from build123d import *

# Parameters (mm, degrees)
ESQUISSE1_W             = 47
ESQUISSE1_H             = 25
BOSS_EXTRU_1_DEPTH      = 5
ESQUISSE2_W             = 4
ESQUISSE2_H             = 4
ENL_V_MAT_EXTRU_1_DEPTH = 5
ESQUISSE4_W             = 47
ESQUISSE4_H             = 12
BOSS_EXTRU_2_DEPTH      = 3
ESQUISSE5_R             = 3
ENL_V_MAT_EXTRU_2_DEPTH = 63


with BuildPart() as part:
    # Esquisse1 → Boss.-Extru.1 (new body)
    with BuildSketch(Plane.XY):
        with Locations((-12.5, -7.5)):
            Rectangle(ESQUISSE1_W, ESQUISSE1_H)
    extrude(amount=BOSS_EXTRU_1_DEPTH)

    # Esquisse2 → Enlèv. mat.-Extru.1 (cut)
    with BuildSketch(Plane.XY.offset(5)):
        with Locations((-25.3, -16)):
            Rectangle(ESQUISSE2_W, ESQUISSE2_H)
        with Locations((-25.3, 1)):
            Rectangle(ESQUISSE2_W, ESQUISSE2_H)
        with Locations((0.3, 1)):
            Rectangle(ESQUISSE2_W, ESQUISSE2_H)
        with Locations((0.3, -16)):
            Rectangle(ESQUISSE2_W, ESQUISSE2_H)
    extrude(amount=-ENL_V_MAT_EXTRU_1_DEPTH, mode=Mode.SUBTRACT)

    # Esquisse4 → Boss.-Extru.2 (add)
    with BuildSketch(Plane.XY.offset(5)):
        with Locations((-12.5, -7.5)):
            Rectangle(ESQUISSE4_W, ESQUISSE4_H)
    extrude(amount=BOSS_EXTRU_2_DEPTH)

    # Esquisse5 → Enlèv. mat.-Extru.2 (cut)
    with BuildSketch(Plane(origin=(11, 0, 0), x_dir=(0, 0, -1), z_dir=(1, 0, 0))):
        with Locations((-8, -7.5)):
            Circle(ESQUISSE5_R)
    extrude(amount=-ENL_V_MAT_EXTRU_2_DEPTH, mode=Mode.SUBTRACT)


solid = part.part
CAD build for the part. Positions are in the model's coordinates, mm. A direction names the side the tool comes from. Round coordinates to 2 decimals unless told otherwise and drop trailing zeros. Loops run counter-clockwise (first coordinate to the right, second up) from the corner with the lowest first, then second, coordinate; pieces in that order, holes last.
(1) Cut at A-A (y = 1). Give the cut face in (x, z).
(2) Cut at C-C (z = 7). Give the cut face in (x, y).
(3) Which spindle directions (+Z, -Z, +X, -X, +Y, -Y) get a long thin tool onto all of the face, cutting with end or side? Do faces 3 (the flat face through (-13, -13.5, 6)), 4 (the flat face through (-13, 2, 5)), 5 (the flat face through (-27.3, -16, 3)). Say none if no direction does.
(4) Cut at D-D (x = 3.5). Give the cut face in (y, z), plus the area to 3 significant figures.
(5) Cut at B-B (z = 1.25). Give the cut face in (x, y), plus the area to 3 significant figures.
(6) Two-plate mould, pull along X, no slides. Class faces 1 (the flat face through (2.3, -16, 3)), 2 (the flat face through (-13, -12, 8)): +X half, -X half, draft (parallel to the pull), parting line (faces both ways), or undercut.
(7) Drop flat-ended pins along their axis: pin 1 (1.5 mm diameter, centred on x = -6.5, z = 6, fed in from +Y); pin 2 (5 mm diameter, centred on x = -8, y = 3, fed in from +Z). Give the stop position or say it passes through.
(8) Wall check: line 1 along X through (y, z) = (2.25, 2.25); line 2 along Z through (x, y) = (7.5, 0); line 3 along Y through (x, z) = (-25, 6). Give the ranges that are in metal, low to high.
Findings below:
1. outline: (-36, 0) - (-27.3, 0) - (-27.3, 5) - (-36, 5) - close; (-23.3, 0) - (-1.7, 0) - (-1.7, 5) - (-23.3, 5) - close; (2.3, 0) - (11, 0) - (11, 5) - (2.3, 5) - close
2. outline: (-36, -13.5) - (11, -13.5) - (11, -10.33) - (-36, -10.33) - close; (-36, -4.67) - (11, -4.67) - (11, -1.5) - (-36, -1.5) - close
3. face 3: +Z, +X, -X, -Y
3. face 4: +Z, +X, -X, +Y
3. face 5: +Z, -Z
4. outline: (-20, 0) - (5, 0) - (5, 5) - (-1.5, 5) - (-1.5, 8) - (-4.5, 8) arc R3 cw to (-10.5, 8) - (-13.5, 8) - (-13.5, 5) - (-20, 5) - close
4. area: 147 mm2
5. outline: (-36, -20) - (11, -20) - (11, 5) - (-36, 5) - close; hole (-27.3, -18) - (-23.3, -18) - (-23.3, -14) - (-27.3, -14) - close; hole (-27.3, -1) - (-23.3, -1) - (-23.3, 3) - (-27.3, 3) - close; hole (-1.7, -18) - (2.3, -18) - (2.3, -14) - (-1.7, -14) - close; hole (-1.7, -1) - (2.3, -1) - (2.3, 3) - (-1.7, 3) - close
5. area: 1,110 mm2
6. face 1: undercut
6. face 2: draft
7. pin 1: stops at y = -1.5
7. pin 2: stops at z = 5
8. line 1: x = -36 to -27.3, -23.3 to -1.7, 2.3 to 11
8. line 2: z = 0 to 5
8. line 3: y = -13.5 to -9.74, -5.26 to -1.5
